Autodesk Inventor part; units mm, degrees
ref_plane "Work Plane1" through (0, 0, 0) normal (0, 0, 1) x (1, 0, 0)
ref_plane "YZ Plane" through (0, 0, 0) normal (1, 0, 0) x (0, 1, 0)
ref_plane "XZ Plane" through (0, 0, 0) normal (0, 1, 0) x (-1, 0, 0)
sketch "Sketch1" plane through (0, 0, 0) normal (0, 1, 0) x (-1, 0, 0)
  circle A0 centre (0, 0) radius 5
  dimension "d0" = 10
extrude "Extrusion1" add sketch "Sketch1" along normal blind 1
ref_plane "Work Plane1" through (0, 0, 0) normal (0, 0, 1) x (1, 0, 0)
sketch "Sketch2" plane through (0, 0, 0) normal (0, 0, 1) x (1, 0, 0)
  line L0 (0, 0) -> (0, 4)
  circle A0 centre (0, 4) radius 1
  circle A1 centre (0, 4) radius 2
  line L1 (5, 1) -> (-5, 1)
  line L2 (0, 1) -> (3.5, 1)
  line L3 (0, 1) -> (-3.5, 1)
  line L4 (-3.5, 1) -> (-1.8315, 4.8034)
  line L5 (3.5, 1) -> (1.8315, 4.8034)
  dimension "d4" = 4
  dimension "d5" = 2
  dimension "d6" = 4
  dimension "d7" = 3.5
  dimension "d8" = 3.5
extrude "Extrusion2" add sketch "Sketch2" along normal mid plane 5
sketch "Sketch3" plane through (0, 0, 0) normal (0, 0, 1) x (1, 0, 0)
  arc A0 (1.8315, 4.8034) -> (-1.8315, 4.8034) centre (0, 4) ccw
  circle A1 centre (0, 4) radius 1
  circle A2 centre (0, 4) radius 2
  line L0 (-1.8315, 4.8034) -> (-3.5, 1)
  line L1 (-1.8315, 4.8034) -> (-3.5, 1)
  line L2 (5, 1) -> (-5, 1)
  line L3 (3.5, 1) -> (1.8315, 4.8034)
  line L4 (1.8315, 4.8034) -> (3.5, 1)
  line L5 (3.5, 1) -> (-3.5, 1)
  point P0 (0, 0)
  dimension "d11" = 4
extrude "Extrusion3" cut sketch "Sketch3" along normal mid plane 2.6 contours A2 A0 | L3 L2 L0 A2 | A1
properties part number "New_Arm_plate"
Check sheet for the modelled part. Datum: model origin and axes. Units: mm. A direction names the side the tool comes from. Coordinates: 2 decimals unless noted, no trailing zeros. Loops run counter-clockwise (first coordinate to the right, second up) from the corner with the lowest first, then second, coordinate; pieces in that order, holes last.
1) Gauge pin test, flat ends, axial feed: pin 1 (1.6 mm diameter, centred on x = 0, y = 4, fed in from +Z); pin 2 (1 mm diameter, centred on x = -4, z = -0.5, fed in from -Y); pin 3 (3 mm diameter, centred on x = 0, y = 4, fed in from -Z); pin 4 (1 mm diameter, centred on y = 3.5, z = 2.5, fed in from +X). Record the tip position at first contact, or that the pin passes through.
2) Sectioned sample at C-C (y = 3.55). Record the boundary of the cut face in (x, z), and give its area (3 significant figures).
3) Release check for a two-part mould opening along Y. For faces 5 (the face through (0, 3, 2)), 6 (the face through (0, 2, 1.3)), 7 (the face through (0, 6, -2)), 8 (the face through (0, 3, -2)) record: released by +Y, released by -Y, zero draft, split by the parting line, or undercut.
4) Sectioned sample at A-A (x = 0). Record the boundary of the cut face in (y, z), and give its area (3 significant figures).
5) Sectioned sample at B-B (y = 1.65). Record the boundary of the cut face in (x, z), and give its area (3 significant figures).
6) Sectioned sample at D-D (z = 0). Record the boundary of the cut face in (x, y), and give its area (3 significant figures).
7) Material ranges on probe 1 along Y at (x, z) = (0, 2); probe 2 along Z at (x, y) = (2, 3.1); probe 3 along Y at (x, z) = (2.25, -1), recorded low to high.
8) Access from +Z, -Z, +X, -X, +Y, -Y to the whole of each face (thin tool, end or side, straight path). Record for faces 1 (the face through (0, 2, -2.5)), 2 (the face through (0, 2, 2.5)), 3 (the face through (0, 6, 2)), 4 (the face through (0, 2, -1.3)).
Check sheet entries:
1. pin 1: passes through
1. pin 2: stops at y = 0
1. pin 3: stops at z = -2.5
1. pin 4: stops at x = 2.62
2. outline: (-2.38, -2.5) - (-0.89, -2.5) - (-0.89, -1.3) - (-2.38, -1.3) - close; (-2.38, 1.3) - (-0.89, 1.3) - (-0.89, 2.5) - (-2.38, 2.5) - close; (0.89, -2.5) - (2.38, -2.5) - (2.38, -1.3) - (0.89, -1.3) - close; (0.89, 1.3) - (2.38, 1.3) - (2.38, 2.5) - (0.89, 2.5) - close
2. area: 7.14 mm2
3. face 5: undercut
3. face 6: zero draft
3. face 7: released by +Y
3. face 8: undercut
4. outline: (0, -5) - (1, -5) - (1, -2.5) - (3, -2.5) - (3, -1.3) - (1, -1.3) - (1, 1.3) - (3, 1.3) - (3, 2.5) - (1, 2.5) - (1, 5) - (0, 5) - close; (5, -2.5) - (6, -2.5) - (6, -1.3) - (5, -1.3) - close; (5, 1.3) - (6, 1.3) - (6, 2.5) - (5, 2.5) - close
4. area: 17.2 mm2
5. outline: (-3.21, -2.5) - (3.21, -2.5) - (3.21, -1.3) - (-3.21, -1.3) - close; (-3.21, 1.3) - (3.21, 1.3) - (3.21, 2.5) - (-3.21, 2.5) - close
5. area: 15.4 mm2
6. outline: (-5, 0) - (5, 0) - (5, 1) - (-5, 1) - close
6. area: 10.0 mm2
7. probe 1: y = 0 to 3, 5 to 6
7. probe 2: z = -2.5 to -1.3, 1.3 to 2.5
7. probe 3: y = 0 to 1
8. face 1: -Z, +X, -X, +Y
8. face 2: +Z, +X, -X, +Y
8. face 3: +Z, -Z, +Y
8. face 4: +X, -X, +Y
